from build123d import *

# Parameters (mm, degrees)
BOSS_EXTRUDE1_DEPTH  = 4
SKETCH2_R            = 2
SKETCH2_R_2          = 1.5
CUT_EXTRUDE1_DEPTH   = 5
BOSS_EXTRUDE5_DEPTH  = 4
SKETCH6_W            = 18
SKETCH6_H            = 34
BOSS_EXTRUDE6_DEPTH  = 4
SKETCH7_W            = 14
SKETCH7_H            = 10
BOSS_EXTRUDE7_DEPTH  = 4
SKETCH8_R            = 2
CUT_EXTRUDE2_DEPTH   = 23
SKETCH9_R            = 2
CUT_EXTRUDE3_DEPTH   = 4
BOSS_EXTRUDE8_DEPTH  = 22
BOSS_EXTRUDE9_DEPTH  = 4
BOSS_EXTRUDE10_DEPTH = 4
CUT_EXTRUDE5_DEPTH   = 4
FILLET7_R            = 2.5
FILLET8_R            = 2.5


with BuildPart() as part:
    # Sketch1 → Boss-Extrude1 (new body)
    with BuildSketch(Plane(origin=(0, 0, 0), x_dir=(1, 0, 0), z_dir=(0, 1, 0))):
        Polygon((-20, 66), (20, 66), (20, 6), (20, 0), (-20, 0), (-20, 6), align=None)
    extrude(amount=BOSS_EXTRUDE1_DEPTH)

    # Sketch2 → Cut-Extrude1 (cut, through all)
    with BuildSketch(Plane(origin=(0, 4, 0), x_dir=(1, 0, 0), z_dir=(0, 1, 0))):
        with Locations((-8.00387182, 61.25)):
            Circle(SKETCH2_R)
        with Locations((1.99612818, 61.25)):
            Circle(SKETCH2_R)
        with Locations((11.99612818, 61.25)):
            Circle(SKETCH2_R)
        with Locations((-5.50387182, 8)):
            Circle(SKETCH2_R)
        with Locations((-5.50387182, 28)):
            Circle(SKETCH2_R)
        with Locations((9.49612818, 28)):
            Circle(SKETCH2_R)
        with Locations((9.49612818, 8)):
            Circle(SKETCH2_R)
        with Locations((15.74612818, 36.25)):
            Circle(SKETCH2_R_2)
        with Locations((15.74612818, 43.75)):
            Circle(SKETCH2_R_2)
        with Locations((-11.75387182, 43.75)):
            Circle(SKETCH2_R_2)
        with Locations((-11.75387182, 36.25)):
            Circle(SKETCH2_R_2)
    extrude(amount=-CUT_EXTRUDE1_DEPTH, mode=Mode.SUBTRACT)

    # Sketch5 → Boss-Extrude5 (add)
    with BuildSketch(Plane(origin=(2, 0, 0), x_dir=(0, 0, -1), z_dir=(1, 0, 0))):
        Polygon((0, 4), (0, 38), (4, 38), (38, 4), align=None)
    extrude(amount=-BOSS_EXTRUDE5_DEPTH)

    # Sketch6 → Boss-Extrude6 (add)
    with BuildSketch(Plane.XY):
        with Locations((-11, 21)):
            Rectangle(SKETCH6_W, SKETCH6_H)
    extrude(amount=-BOSS_EXTRUDE6_DEPTH)

    # Sketch7 → Boss-Extrude7 (add)
    with BuildSketch(Plane.XY):
        with Locations((13, 9)):
            Rectangle(SKETCH7_W, SKETCH7_H)
    extrude(amount=-BOSS_EXTRUDE7_DEPTH)

    # Sketch8 → Cut-Extrude2 (cut, through all)
    with BuildSketch(Plane.ZY.offset(2)):
        with Locations((-10, 24)):
            Circle(SKETCH8_R)
        with Locations((-22, 12)):
            Circle(SKETCH8_R)
    extrude(amount=-CUT_EXTRUDE2_DEPTH, mode=Mode.SUBTRACT)

    # Sketch9 → Cut-Extrude3 (cut)
    with BuildSketch(Plane(origin=(0, 0, -4), x_dir=(-1, 0, 0), z_dir=(0, 0, -1))):
        with Locations((10, 12)):
            Circle(SKETCH9_R)
        with Locations((10, 30)):
            Circle(SKETCH9_R)
    extrude(amount=-CUT_EXTRUDE3_DEPTH, mode=Mode.SUBTRACT)

    # Sketch10 → Boss-Extrude8 (add)
    with BuildSketch(Plane(origin=(2, 0, 0), x_dir=(0, 0, -1), z_dir=(1, 0, 0))):
        Polygon((4, 38), (0, 42), (0, 38), align=None)
    extrude(amount=-BOSS_EXTRUDE8_DEPTH)

    # Sketch13 → Boss-Extrude9 (add)
    with BuildSketch(Plane(origin=(20, 0, 0), x_dir=(0, 0, -1), z_dir=(1, 0, 0))):
        Polygon((4, 14), (14, 4), (4, 4), align=None)
    extrude(amount=-BOSS_EXTRUDE9_DEPTH)

    # Sketch14 → Boss-Extrude10 (add)
    with BuildSketch(Plane.ZY.offset(20)):
        Polygon((-4, 38), (-38, 4), (-4, 4), align=None)
    extrude(amount=-BOSS_EXTRUDE10_DEPTH)

    # Sketch16 → Cut-Extrude5 (cut)
    with BuildSketch(Plane.XY):
        with BuildLine():
            Line((-20, 42), (-20, 39.566764618))
            ThreePointArc((-20, 39.566764618), (-19.278186488, 41.259842846), (-17.593046725, 42))
            Line((-17.593046725, 42), (-20, 42))
        make_face()
    extrude(amount=-CUT_EXTRUDE5_DEPTH, mode=Mode.SUBTRACT)

    # Fillet7
    fillet7_edges = [part.edges().sort_by_distance(p)[0] for p in [
        (-20, 2, -66),
        (20, 2, -66),
    ]]
    fillet(fillet7_edges, radius=FILLET7_R)

    # Fillet8
    fillet8_edges = [part.edges().sort_by_distance(p)[0] for p in [
        (20, 14, -2),
    ]]
    fillet(fillet8_edges, radius=FILLET8_R)


solid = part.part
Source: CAD feature listing. Evaluate the final solid. Frame: model axes, mm. A direction names the side the tool comes from. Round coordinates to 2 decimals unless told otherwise and drop trailing zeros. Loops run counter-clockwise (first coordinate to the right, second up) from the corner with the lowest first, then second, coordinate; pieces in that order, holes last. Notation, with made-up numbers: (-21.5, 33) - (37.5, 33) arc R26 ccw to (37.5, 48) - close; hole circle Ø2 at (27.25, -14.5). An arc over 180 degrees is marked (long way). Write item = value, one per line. Start each with the question number.
(1) Pull-direction query (X, two-part tool) for faces 4 (the face through (-19.77, 40.55, -0.66)), 5 (the face through (-9, 21, -4)), 6 (the face through (0, 2, -66)); classes: +X half, -X half, draft (parallel to the pull), parting line (faces both ways), or undercut.
(2) Set-up query: faces 1 (the face through (18, 9, -9)), 2 (the face through (-16, 14, -14)), 3 (the face through (0, 22.8, -11.6)). Return all of +Z, -Z, +X, -X, +Y, -Y with unobstructed straight access to the full face (end or side cutting, diameter ignored); none if empty.
(3) Section query C-C, the plane y = 24. Output: boundary loops of the cut face in (x, z).
(4) Section query B-B, the plane x = -5. Output: boundary loops of the cut face in (y, z), plus the area to 3 significant figures.
(5) Section query A-A, the plane z = -28. Output: boundary loops of the cut face in (x, y).
(6) Section query D-D, the plane z = -43.75. Output: boundary loops of the cut face in (x, y).
(7) Pin query (flat end, axial travel): pin 1 (12 mm diameter, centred on y = 12.5, z = -44.5, fed in from +X); pin 2 (7 mm diameter, centred on x = -9, y = 25.5, fed in from -Z); pin 3 (6 mm diameter, centred on x = -0.5, z = -39.5, fed in from +Y); pin 4 (3 mm diameter, centred on x = 11.5, z = -2, fed in from +Y). Return the tip coordinate at first contact, or that it passes through.
(8) Ray query, line 1 along X through (y, z) = (0.8, -61.25); line 2 along Y through (x, z) = (-10, -2.85); line 3 along X through (y, z) = (21.5, -7). Return the intervals inside material, ascending. Write a range as from..to.
Conclusion:
q1.face_4 = -X half
q1.face_5 = undercut
q1.face_6 = draft
q2.face_1 = -Z, +X, +Y
q2.face_2 = -Z, +Y
q2.face_3 = +X
q3.outline = (-20, -18) - (-16, -18) - (-16, -4) - (-2, -4) - (-2, -8) - (2, -8) - (2, 0) - (-20, 0) - close; (-2, -18) - (2, -18) - (2, -12) - (-2, -12) - close
q4.outline = (0, -66) - (4, -66) - (4, -29.94) - (0, -29.94) - close; (0, -26.06) - (4, -26.06) - (4, -9.94) - (0, -9.94) - close; (0, -6.06) - (4, -6.06) - (4, -4) - (38, -4) - (42, 0) - (0, 0) - close
q4.area = 377 mm2
q5.outline = (-20, 0) - (-7.5, 0) - (-7.5, 4) - (-16, 4) - (-16, 14) - (-20, 14) - close; (-3.5, 0) - (7.5, 0) - (7.5, 4) - (2, 4) - (2, 14) - (-2, 14) - (-2, 4) - (-3.5, 4) - close; (11.5, 0) - (20, 0) - (20, 4) - (11.5, 4) - close
q6.outline = (-20, 0) - (-13.25, 0) - (-13.25, 4) - (-20, 4) - close; (-10.25, 0) - (14.25, 0) - (14.25, 4) - (-10.25, 4) - close; (17.25, 0) - (20, 0) - (20, 4) - (17.25, 4) - close
q7.pin_1 = through
q7.pin_2 = -4
q7.pin_3 = 5.5
q7.pin_4 = 14
q8.line_1 = -20..-10, -6..0, 4..10, 14..20
q8.line_2 = 0..10, 14..28, 32..39.15
q8.line_3 = -20..-16, -2..2
